Design review of the part built by this model. Coordinates are the model's own, in mm. A direction names the side the tool comes from. Coordinates: 2 decimals unless noted, no trailing zeros. Write each loop counter-clockwise with the first axis right and the second up, starting at its lowest first coordinate (ties: lowest second). Pieces come first, ordered by that corner, then holes. Notation, with made-up numbers: (65.25, 87.25) -> (124.25, 87.25) arc R8 cw to (124.25, 99.25) -> close; hole circle Ø4 at (57.25, 75.25). An arc over 180 degrees is marked (long way). Write item = value, one per line. Start each with the question number.
```python
from build123d import *

# Parameters (mm, degrees)
SKETCH4_R           = 10
SKETCH4_R_2         = 2
BOSS_EXTRUDE4_DEPTH = 3
SKETCH5_R           = 1.75
CUT_EXTRUDE1_DEPTH  = 10.25
SKETCH7_R           = 3
CUT_EXTRUDE3_DEPTH  = 2
CUT_EXTRUDE2_DEPTH  = 10.25


with BuildPart() as part:
    # Sketch3 → Revolve1 (revolve)
    with BuildSketch(Plane(origin=(0, 0, 0), x_dir=(0, 0, -1), z_dir=(1, 0, 0))):
        Polygon((0, 2), (0, 2.746804147), (-6.25, 2.2), (-6.25, 2), align=None)
    revolve(axis=Axis((0, 0, 0), (0, 0, 1)))

    # Sketch4 → Boss-Extrude4 (add)
    with BuildSketch(Plane(origin=(0, 0, 0), x_dir=(-1, 0, 0), z_dir=(0, 0, -1))):
        Circle(SKETCH4_R)
        Circle(SKETCH4_R_2, mode=Mode.SUBTRACT)
    extrude(amount=BOSS_EXTRUDE4_DEPTH)

    # Sketch5 → Cut-Extrude1 (cut, through all)
    with BuildSketch(Plane(origin=(0, 0, -3), x_dir=(-1, 0, 0), z_dir=(0, 0, -1))):
        with Locations((0, 6)):
            Circle(SKETCH5_R)
        with Locations((-5.196152423, -3)):
            Circle(SKETCH5_R)
        with Locations((5.196152423, -3)):
            Circle(SKETCH5_R)
    extrude(amount=-CUT_EXTRUDE1_DEPTH, mode=Mode.SUBTRACT)

    # Sketch7 → Cut-Extrude3 (cut)
    with BuildSketch(Plane(origin=(0, 0, -3), x_dir=(-1, 0, 0), z_dir=(0, 0, -1))):
        with Locations((0, 6)):
            Circle(SKETCH7_R)
        with Locations((5.196152423, -3)):
            Circle(SKETCH7_R)
        with Locations((-5.196152423, -3)):
            Circle(SKETCH7_R)
    extrude(amount=-CUT_EXTRUDE3_DEPTH, mode=Mode.SUBTRACT)

    # Sketch6 → Cut-Extrude2 (cut, through all)
    with BuildSketch(Plane(origin=(0, 0, -3), x_dir=(-1, 0, 0), z_dir=(0, 0, -1))):
        with BuildLine():
            Line((-8.829948007, 4.69382767), (-0.175, -0.303108891))
            Line((-0.175, -0.303108891), (0, 0))
            Line((0, 0), (0.175, 0.303108891))
            Line((0.175, 0.303108891), (-8.479948007, 5.300045453))
            ThreePointArc((-8.479948007, 5.300045453), (-8.660254038, 5), (-8.829948007, 4.69382767))
        make_face()
    extrude(amount=-CUT_EXTRUDE2_DEPTH, mode=Mode.SUBTRACT)


solid = part.part
```
(1) For faces 4 (the face through (-2.1, -2.1, 0)), 5 (the face through (-2, 6, -1)), 6 (the face through (5.404, 2.716, -1.523)), list the 3-axis set-ups (+Z, -Z, +X, -X, +Y, -Y) from which the entire face can be reached by the end or side of a thin tool; tool diameter is ignored.
(2) For pin 1 Ø5 at (x, y) = (5.2, -3) entering from -Z; pin 2 Ø3 at (y, z) = (-5, -1) entering from -X; pin 3 Ø3 at (y, z) = (2, 3) entering from +X, all flat-tipped, find the tip position at first contact; note any pin that passes through.
(3) Mouldability with a two-part tool opening along X and no side actions: class faces 1 (the face through (4.184, 2.82, -1.523)), 2 (the face through (-2, -2, -3)), 3 (the face through (-2.19, -1.14, 3.17)) as pulls with the +X half, pulls with the -X half, needs draft (parallel to the pull), parting line crosses it, or undercut.
(4) For line 1 (Y direction, x = 0, z = -0.3); line 2 (Z direction, x = 3.5, y = -1.25); line 3 (Z direction, x = -3, y = -6.75), list the stretches that pass through material, from the lowest coordinate up.
(5) Take a section at A-A, the plane y = 6. State the section outline as (x, z) points.
(6) Take a section at C-C, the plane z = -0.5. State the section outline as (x, y) points.
(7) Take a section at D-D, the plane x = -4. State the section outline as (y, z) points, then the cut area to 3 significant figures.
(8) Take a section at B-B, the plane x = 0. State the section outline as (y, z) points.
Report:
q1.face_4 = +Z
q1.face_5 = -Z
q1.face_6 = +Z, -Z
q2.pin_1 = -1
q2.pin_2 = -9.37
q2.pin_3 = 2.46
q3.face_1 = undercut
q3.face_2 = needs draft
q3.face_3 = parting line crosses it
q4.line_1 = -10 to -2, 2 to 4.25, 7.75 to 10
q4.line_2 = -1 to 0
q4.line_3 = -3 to 0
q5.outline = (-8, -3) -> (-3, -3) -> (-3, -1) -> (-1.75, -1) -> (-1.75, 0) -> (-8, 0) -> close; (1.75, -1) -> (3, -1) -> (3, -3) -> (8, -3) -> (8, 0) -> (1.75, 0) -> close
q6.outline = (1.53, 1.29) -> (8.48, 5.3) arc R10 ccw (long way) to (8.83, 4.69) -> (1.88, 0.68) arc R2 cw (long way) to start; hole circle Ø3.5 at (-5.2, -3); hole circle Ø3.5 at (0, 6); hole circle Ø3.5 at (5.2, -3)
q7.outline = (-9.17, -3) -> (-5.75, -3) -> (-5.75, -1) -> (-4.28, -1) -> (-4.28, 0) -> (-9.17, 0) -> close; (-1.72, -1) -> (-0.25, -1) -> (-0.25, -3) -> (9.17, -3) -> (9.17, 0) -> (-1.72, 0) -> close
q7.area = 41.4 mm2
q8.outline = (-10, -3) -> (-2, -3) -> (-2, 6.25) -> (-2.2, 6.25) -> (-2.75, 0) -> (-10, 0) -> close; (2, -3) -> (3, -3) -> (3, -1) -> (4.25, -1) -> (4.25, 0) -> (2.75, 0) -> (2.2, 6.25) -> (2, 6.25) -> close; (7.75, -1) -> (9, -1) -> (9, -3) -> (10, -3) -> (10, 0) -> (7.75, 0) -> close
